The listing builds one solid part. Answer for the finished solid, in the listing's coordinates (mm). Face numbers are marked on the shaded views. A direction names the side the tool comes from. Coordinates: 2 decimals unless noted, no trailing zeros. Order: outer loops, then holes, each group sorted by start corner. A loop starts at its lowest first (then second) coordinate and runs counter-clockwise, first axis right, second up. Notation, with made-up numbers: (-15.75, 17.25) - (8.25, 17.25) arc R26 ccw to (8.25, 39.25) - close; hole circle Ø5 at (-7, 25). An arc over 180 degrees is marked (long way). Use one line per item in the form item = value. Start each with the question number.
Item 1: Each of these flat-tipped pins is pushed along its axis until it touches: pin 1 Ø8.5 at (y, z) = (0.5, 14.5) entering from +X (3 decimals); pin 2 Ø2.5 at (y, z) = (0.5, 13) entering from -X (3 decimals); pin 3 Ø8 at (y, z) = (9, 7.5) entering from +X. Where does it stop, or does it pass through?
Item 2: Section B-B, the plane y = 0 is taken. Write down the section's boundary in (x, z) (1 decimal), and give its area (3 significant figures).
Item 3: Section C-C, the plane z = 14.75 is taken. Write down the section's boundary in (x, y) (1 decimal), and give its area (3 significant figures).
Item 4: Consider line 1 along Y through (x, z) = (0, 12); line 2 along X through (y, z) = (4.25, 8); line 3 along X through (y, z) = (3.5, 10.5) (3 decimals). Determine where each line is inside the solid, lowest interval first. Write a range as [from, to].
Item 5: The mould has two halves that part along Y. Classify the marked faces 3, 4 and 5: released by +Y, released by -Y, zero draft, split by the parting line, or undercut.
Item 6: Section A-A, the plane x = 0 is taken. Write down the section's boundary in (y, z), and give its area (3 significant figures).
Item 7: Section D-D, the plane x = -4.25 is taken. Write down the section's boundary in (y, z).
Item 8: A tool of negligible diameter and unlimited length cuts with its end or side. For the marked faces 1 and 2, from which of +Z, -Z, +X, -X, +Y, -Y can it reach the whole face along a straight path? Write none if from no direction.
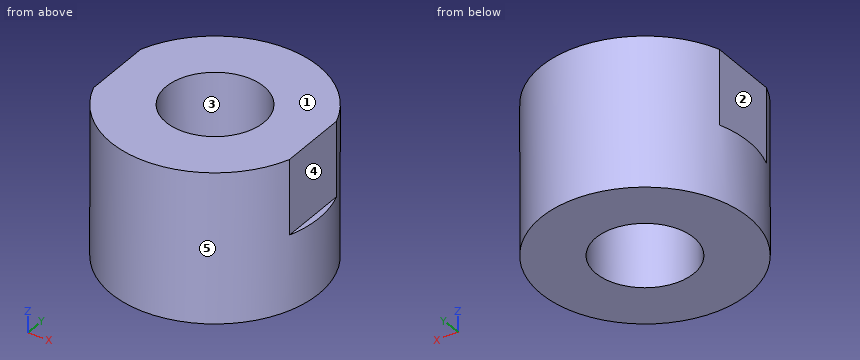
Autodesk Inventor part; units mm, degrees
ref_plane "YZ Plane" through (0, 0, 0) normal (1, 0, 0) x (0, 1, 0)
ref_plane "XZ Plane" through (0, 0, 0) normal (0, 1, 0) x (-1, 0, 0)
ref_plane "XY Plane" through (0, 0, 0) normal (0, 0, 1) x (1, 0, 0)
sketch "Sketch1" plane through (0, 0, 0) normal (0, 0, 1) x (1, 0, 0)
  circle A0 centre (0, 0) radius 11.4681
  circle A1 centre (0, 0) radius 5.3975
  dimension "d0" = 10.795
  dimension "d1" = 22.9362
extrude "Extrusion1" add sketch "Sketch1" along normal blind 8.255
sketch "Sketch2" plane through (0, 0, 8.255) normal (0, 0, 1) x (1, 0, 0)
  circle A0 centre (0, 0) radius 5.3975
  circle A1 centre (0, 0) radius 11.4681
  circle A2 centre (0, 0) radius 11.4681
  line L0 (-10.795, 3.8711) -> (-10.795, -3.8711)
  line L1 (10.795, 3.8711) -> (10.795, -3.8711)
  dimension "d4" = 21.59
extrude "Extrusion2" add sketch "Sketch2" along normal blind 8.255 contours L1 A1 L0
properties part number "Suction Cup Part 3 1764"
Response:
q1.pin_1 = 10.795
q1.pin_2 = -10.795
q1.pin_3 = 10.32
q2.outline = (-11.5, 0) - (-5.4, 0) - (-5.4, 16.5) - (-10.8, 16.5) - (-10.8, 8.3) - (-11.5, 8.3) - close; (5.4, 0) - (11.5, 0) - (11.5, 8.3) - (10.8, 8.3) - (10.8, 16.5) - (5.4, 16.5) - close
q2.area = 189 mm2
q3.outline = (-10.8, -3.9) arc R11.5 ccw to (10.8, -3.9) - (10.8, 3.9) arc R11.5 ccw to (-10.8, 3.9) - close; hole circle Ø10.8 at (0, 0)
q3.area = 315 mm2
q4.line_1 = [-11.47, -5.4], [5.4, 11.47]
q4.line_2 = [-10.65, -3.33], [3.33, 10.65]
q4.line_3 = [-10.795, -4.109], [4.109, 10.795]
q5.face_3 = undercut
q5.face_4 = zero draft
q5.face_5 = split by the parting line
q6.outline = (-11.47, 0) - (-5.4, 0) - (-5.4, 16.51) - (-11.47, 16.51) - close; (5.4, 0) - (11.47, 0) - (11.47, 16.51) - (5.4, 16.51) - close
q6.area = 200 mm2
q7.outline = (-10.65, 0) - (-3.33, 0) - (-3.33, 16.51) - (-10.65, 16.51) - close; (3.33, 0) - (10.65, 0) - (10.65, 16.51) - (3.33, 16.51) - close
q8.face_1 = +Z, +X, -X, +Y, -Y
q8.face_2 = +Z, -X, +Y, -Y
